Design review of the part shown in the three views and the two pictorial views. Dimensions are in mm from the part's minimum x, y and z. A direction names the side the tool comes from. Round coordinates to 2 decimals unless told otherwise and drop trailing zeros. Write each loop counter-clockwise with the first axis right and the second up, starting at its lowest first coordinate (ties: lowest second). Pieces come first, ordered by that corner, then holes. Notation, with made-up numbers: (-26.5, 40.25) -> (18.5, 40.25) arc R29 ccw to (18.5, 72.25) -> close; hole circle Ø9 at (84.25, 69.5). An arc over 180 degrees is marked (long way). One line per question, with ' | ' between items. Start each with the question number.
1) For the marked faces 3 and 4, list the 3-axis set-ups (+Z, -Z, +X, -X, +Y, -Y) from which the entire face can be reached by the end or side of a thin tool; tool diameter is ignored.
2) Insertion check: pin 1 Ø1 at (y, z) = (2, 1) entering from -X; pin 2 Ø2 at (y, z) = (0.5, 0.5) entering from +X; pin 3 Ø1 at (x, y) = (25, 3) entering from +Z. Each pin has a flat end and moves straight along its axis. Give the tip position at first contact, or say it passes through.
3) Consider section C-C (z = 3.1). Give the boundary of the cut face in (x, y).
4) Consider section A-A (x = 2.5). Give the boundary of the cut face in (y, z) (3 decimals), then the cut area to 3 significant figures.
5) For probe 1 along X at (y, z) = (3.85, 2.4); probe 2 along Z at (x, y) = (2.5, 3) (3 decimals); probe 3 along Z at (x, y) = (8.25, 3.8), list the stretches that pass through material, from the lowest coordinate up.
6) Mouldability with a two-part tool opening along X and no side actions: class the marked faces 1 and 2 as +X half, -X half, draft (parallel to the pull), parting line (faces both ways), or undercut.
7) Consider section D-D (x = 27.5). Give the boundary of the cut face in (y, z) (3 decimals), then the cut area to 3 significant figures.
8) Consider section B-B (y = 3.7). Give the boundary of the cut face in (x, z) (3 decimals).
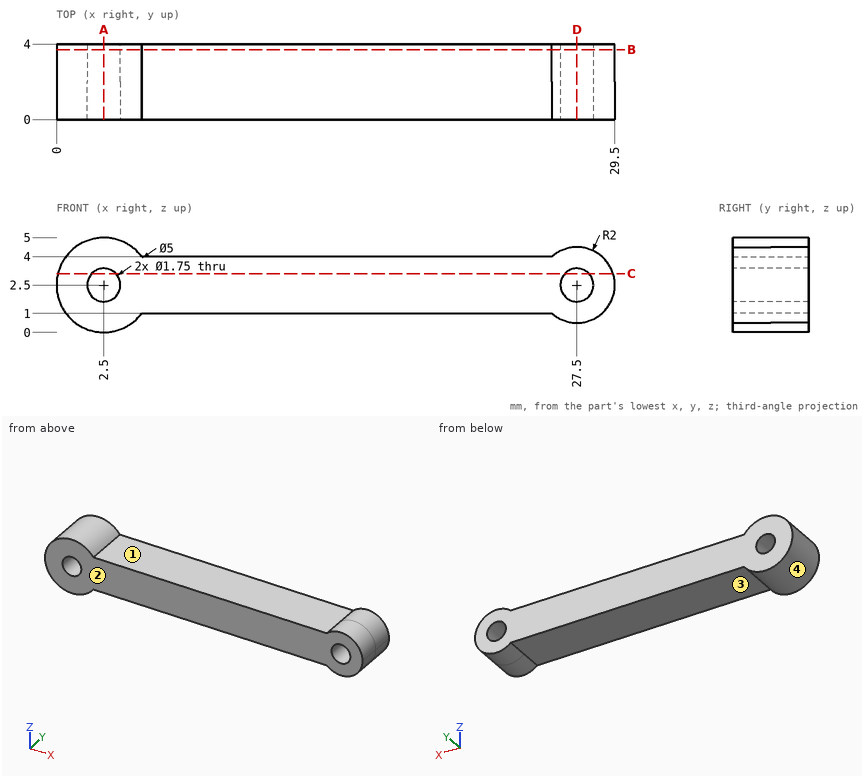
From the geometry:
1) face 3: -Z, +Y, -Y | face 4: +Y, -Y
2) pin 1: stops at x = 0.21 | pin 2: stops at x = 29.23 | pin 3: stops at z = 4
3) outline: (0.07, 0) -> (1.86, 0) -> (1.86, 4) -> (0.07, 4) -> close; (3.14, 0) -> (26.86, 0) -> (26.86, 4) -> (3.14, 4) -> close; (28.14, 0) -> (29.41, 0) -> (29.41, 4) -> (28.14, 4) -> close
4) outline: (0, 0) -> (4, 0) -> (4, 1.625) -> (0, 1.625) -> close; (0, 3.375) -> (4, 3.375) -> (4, 5) -> (0, 5) -> close | area: 13.0 mm2
5) probe 1: x = 0 to 1.63, 3.37 to 26.63, 28.37 to 29.5 | probe 2: z = 0 to 1.625, 3.375 to 5 | probe 3: z = 1 to 4
6) face 1: undercut | face 2: draft
7) outline: (0, 0.5) -> (4, 0.5) -> (4, 1.625) -> (0, 1.625) -> close; (0, 3.375) -> (4, 3.375) -> (4, 4.5) -> (0, 4.5) -> close | area: 9.00 mm2
8) outline: (4.5, 1) -> (26.177, 1) arc R2 ccw (long way) to (26.177, 4) -> (4.5, 4) arc R2.5 ccw (long way) to start; hole circle Ø1.75 at (2.5, 2.5); hole circle Ø1.75 at (27.5, 2.5)
